Check sheet for the modelled part. Datum: model origin and axes. Units: mm. Face numbers are marked on the shaded views. A direction names the side the tool comes from. Give positions to 0.01 mm unless a question says otherwise; leave off trailing zeros. Loops run counter-clockwise (first coordinate to the right, second up) from the corner with the lowest first, then second, coordinate; pieces in that order, holes last. Notation, with made-up numbers: M 13.25,73 L 27.25,73 A30 cw 27.25,102 Z; hole C 27.25,74.5 d9. An arc over 180 degrees is marked long. Write each question's results on one line, items separated by ' | '. Start each with the question number.
1. Draft check along Z on the marked faces 1, 2 and 3. Enter one of: pulls with the +Z half, pulls with the -Z half, needs draft (parallel to the pull), parting line crosses it, or undercut.
2. Tool access check on the marked faces 4, 5, 6, 7 and 8. Record the directions out of +Z, -Z, +X, -X, +Y, -Y that give a thin tool (end or side, any length) a straight path to the whole face; none if there is none.
3. Material ranges on line 1 along Y through (x, z) = (0, 3); line 2 along Z through (x, y) = (18.75, 4); line 3 along Y through (x, z) = (22, 7), recorded low to high.
4. Sectioned sample at D-D on y = 1.75. Record the cut outline in (x, z).
5. Sectioned sample at A-A on x = 0. Record the cut outline in (y, z).
6. Go/stop test with flat-tipped pins: pin 1 (3 mm diameter, centred on x = 18, z = 3, fed in from -Y) (3 decimals); pin 2 (1.7 mm diameter, centred on x = 12, z = 4, fed in from +Y) (3 decimals); pin 3 (4 mm diameter, centred on y = -4.5, z = 4, fed in from +X); pin 4 (1 mm diameter, centred on x = 17.5, z = 3, fed in from -Y). Record where each tip stops, or that it passes through.
7. Sectioned sample at C-C on z = 6.5. Record the cut outline in (x, y).
8. Sectioned sample at B-B on y = 0. Record the cut outline in (x, z), and give its area (3 significant figures).
```python
from build123d import *

# Parameters (mm, degrees)
CYLINDER003006_R               = 2.25
CYLINDER003006_DEPTH           = 11
CYLINDER003005_R               = 3.15
CYLINDER003005_DEPTH           = 8.8181
PAD_DEPTH                      = 1.35
CYLINDER003004_W               = 25
CYLINDER003004_H               = 3
CYLINDER003004_ANGLE           = 30
CYLINDER003004_PLACEMENT_ANGLE = -15


with BuildPart() as obj1:
    # Cylinder003006 → Cylinder003006 (new body)
    with BuildSketch(Plane.XY.offset(-1)):
        Circle(CYLINDER003006_R)
    extrude(amount=CYLINDER003006_DEPTH)


with BuildPart() as exterior_cilindro_central:
    # Cylinder003005 → Cylinder003005 (new body)
    with BuildSketch(Plane.XY):
        Circle(CYLINDER003005_R)
    extrude(amount=CYLINDER003005_DEPTH)


with BuildPart() as obj2:
    # Sketch → Pad (new body)
    with BuildSketch(Plane(origin=(2.12, 0.675, 0), x_dir=(1, 0, 0), z_dir=(0, -1, 0))):
        Polygon((0, -0.084088), (22.85, 5.734012), (0, 5.734012), align=None)
    extrude(amount=PAD_DEPTH)


with BuildPart() as obj3:
    # Cylinder003004 → Cylinder003004 (revolve)
    with BuildSketch(Plane.XZ):
        with Locations((12.5, 1.5)):
            Rectangle(CYLINDER003004_W, CYLINDER003004_H)
    revolve(axis=Axis((0, 0, 0), (0, 0, 1)), revolution_arc=CYLINDER003004_ANGLE)


with BuildPart() as obj3_1:
    # Cylinder003004 placement: moved
    add(obj3.part.moved(Location((0, 0, 5.8181))).rotate(Axis((0, 0, 5.8181), (0, 0, 1)), CYLINDER003004_PLACEMENT_ANGLE))

    # Fusion009: union Exterior  cilindro central, obj2
    add(exterior_cilindro_central.part)
    add(obj2.part)

    # Cut013: cut obj1
    add(obj1.part, mode=Mode.SUBTRACT)


solid = obj3_1.part
```
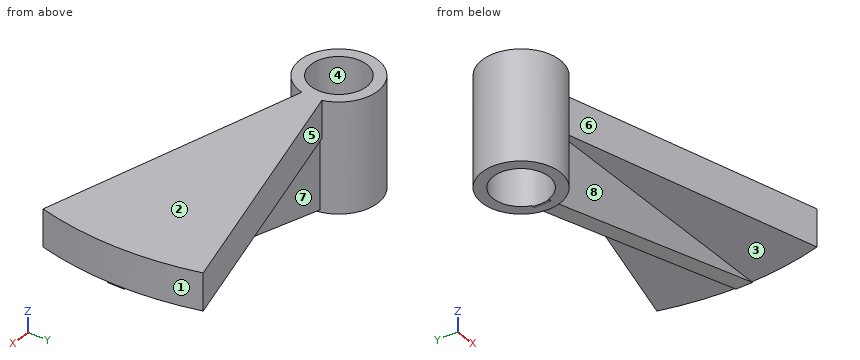
Output values:
1) face 1: needs draft | face 2: pulls with the +Z half | face 3: undercut
2) face 4: +Z, -Z | face 5: +Z, -Z, +Y | face 6: +Z, -Z, -Y | face 7: -Z, +X, +Y | face 8: -Z, +X, -Y
3) line 1: -3.15 to -2.25, 2.25 to 3.15 | line 2: 5.82 to 8.82 | line 3: -5.89 to 5.89
4) outline: M -2.62,0 L -1.41,0 L -1.41,8.82 L -2.62,8.82 Z; M 1.41,0 L 2.62,0 L 2.62,8.82 L 1.41,8.82 Z; M 6.53,5.82 L 24.94,5.82 L 24.94,8.82 L 6.53,8.82 Z
5) outline: M -3.15,0 L -2.25,0 L -2.25,8.82 L -3.15,8.82 Z; M 2.25,0 L 3.15,0 L 3.15,8.82 L 2.25,8.82 Z
6) pin 1: y = -0.675 | pin 2: y = 0.675 | pin 3: x = 24.73 | pin 4: through
7) outline: M 3.04,-0.82 L 24.15,-6.47 A25 ccw 24.15,6.47 L 3.04,0.82 A3.15 ccw long Z; hole C 0,0 d4.5
8) outline: M -3.15,0 L -2.25,0 L -2.25,8.82 L -3.15,8.82 Z; M 2.25,-0.05 L 2.45,0 L 3.15,0 L 3.15,0.18 L 24.97,5.73 L 3.15,5.73 L 3.15,5.82 L 25,5.82 L 25,8.82 L 2.25,8.82 Z | area: 142 mm2
